Can you work these out from the model? Positions are in its coordinate system, mm. Face numbers are marked on the shaded views. A direction names the side the tool comes from. Give positions to 0.01 mm unless a question says otherwise; leave off trailing zeros. Order: outer loops, then holes, each group sorted by start corner. A loop starts at its lowest first (then second) coordinate and runs counter-clockwise, first axis right, second up. Notation, with made-up numbers: (9.25, 65.25) -> (49.25, 65.25) arc R18 cw to (49.25, 72.25) -> close; hole circle Ø4 at (89, -40). An arc over 180 degrees is marked (long way). Answer as CSV lines item,"result".
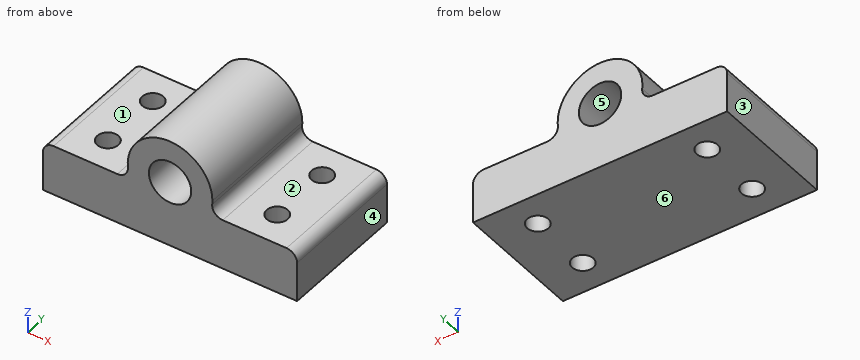
```python
from build123d import *

# Parameters (mm, degrees)
F0_R     = 25.4
F1_DEPTH = 152.4
F2_R     = 12.7
F3_DEPTH = 60.345965


with BuildPart() as f1:
    # F0 (on Front) → F1 (new body)
    with BuildSketch(Plane.XZ):
        with BuildLine():
            ThreePointArc((-50.585668, -4.661564), (-53.848843, -14.385271), (-63.232085, -18.526955))
            Line((-63.232085, -18.526955), (-139.7, -18.526955))
            ThreePointArc((-139.7, -18.526955), (-148.680256, -22.246699), (-152.4, -31.226955))
            Line((-152.4, -31.226955), (-152.4, -78.871921))
            Line((-152.4, -78.871921), (152.4, -78.871921))
            Line((152.4, -78.871921), (152.4, -31.226955))
            ThreePointArc((152.4, -31.226955), (148.680256, -22.246699), (139.7, -18.526955))
            Line((139.7, -18.526955), (63.232085, -18.526955))
            ThreePointArc((63.232085, -18.526955), (53.848843, -14.385271), (50.585668, -4.661564))
            ThreePointArc((50.585668, -4.661564), (0, -50.8), (-50.585668, -4.661564))
        make_face()
        with BuildLine():
            ThreePointArc((50.8, 0), (-2.333245, 50.746389), (-50.585668, -4.661564))
            ThreePointArc((-50.585668, -4.661564), (0, -50.8), (50.585668, -4.661564))
            ThreePointArc((50.585668, -4.661564), (50.746389, -2.333245), (50.8, 0))
        make_face()
        Circle(F0_R, mode=Mode.SUBTRACT)
    extrude(amount=F1_DEPTH)

    # F2 (on face) → F3 (cut, through all)
    with BuildSketch(Plane.XY.offset(-18.526955)):
        with Locations((-101.6, -38.1)):
            Circle(F2_R)
        with Locations((-101.6, -114.3)):
            Circle(F2_R)
        with Locations((101.6, -114.3)):
            Circle(F2_R)
        with Locations((101.6, -38.1)):
            Circle(F2_R)
    extrude(amount=-F3_DEPTH, mode=Mode.SUBTRACT)


solid = f1.part
```
Item 1: We'd pull the mould along Z, two halves only. Please class the marked faces 4, 5 and 6: released by +Z, released by -Z, zero draft, split by the parting line, or undercut.
Numbers:
face 4,"zero draft"
face 5,"undercut"
face 6,"released by -Z"
Item 2: Imagine slicing it at C-C, the plane x = -10.5. Please give me the cut outline in (y, z), then the cut area to 3 significant figures.
Numbers:
outline,"(-152.4, -78.87) -> (0, -78.87) -> (0, -23.13) -> (-152.4, -23.13) -> close; (-152.4, 23.13) -> (0, 23.13) -> (0, 49.7) -> (-152.4, 49.7) -> close"
area,"12,500 mm²"
Item 3: Imagine slicing it at D-D, the plane z = 6. Please give me the cut outline in (x, y).
Numbers:
outline,"(-50.44, -152.4) -> (-24.68, -152.4) -> (-24.68, 0) -> (-50.44, 0) -> close; (24.68, -152.4) -> (50.44, -152.4) -> (50.44, 0) -> (24.68, 0) -> close"
Item 4: Imagine slicing it at A-A, the plane x = -101.6. Please give me the cut outline in (y, z).
Numbers:
outline,"(-152.4, -78.87) -> (-127, -78.87) -> (-127, -18.53) -> (-152.4, -18.53) -> close; (-101.6, -78.87) -> (-50.8, -78.87) -> (-50.8, -18.53) -> (-101.6, -18.53) -> close; (-25.4, -78.87) -> (0, -78.87) -> (0, -18.53) -> (-25.4, -18.53) -> close"
Item 5: Please list where these lines run through material, in increasing order: line 1 along Y through (x, z) = (-101, -63); line 2 along Z through (x, y) = (0, -95); line 3 along Z through (x, y) = (-117, -145.5).
Numbers:
line 1,"y = -152.4 to -126.99, -101.61 to -50.79, -25.41 to 0"
line 2,"z = -78.87 to -25.4, 25.4 to 50.8"
line 3,"z = -78.87 to -18.53"
Item 6: For pin 1 (5 mm diameter, centred on x = 112.5, y = -122, fed in from +Z); pin 2 (12 mm diameter, centred on x = -49.5, y = -47, fed in from +Z); pin 3 (12 mm diameter, centred on y = -26, z = 21.5, fed in from -X), each with a flat end and sliding along its axis, tell me the tip position at first contact or that it passes through.
Numbers:
pin 1,"stops at z = -18.53"
pin 2,"stops at z = 26.24"
pin 3,"stops at x = -48.38"
Item 7: For the marked faces 1, 2 and 3, which set-ups out of +Z, -Z, +X, -X, +Y, -Y let a thin tool reach every point of the face, with its end or its side?
Numbers:
face 1,"+Z, -X, +Y, -Y"
face 2,"+Z, +X, +Y, -Y"
face 3,"+Z, -Z, -X, +Y, -Y"
Item 8: Imagine slicing it at B-B, the plane y = -38.1. Please give me the cut outline in (x, z).
Numbers:
outline,"(-152.4, -78.87) -> (-114.3, -78.87) -> (-114.3, -18.53) -> (-139.7, -18.53) arc R12.7 ccw to (-152.4, -31.23) -> close; (-88.9, -78.87) -> (88.9, -78.87) -> (88.9, -18.53) -> (63.23, -18.53) arc R12.7 cw to (50.59, -4.66) arc R50.8 ccw to (50.8, 0) arc R50.8 ccw (long way) to (-50.59, -4.66) arc R12.7 cw to (-63.23, -18.53) -> (-88.9, -18.53) -> close; (114.3, -78.87) -> (152.4, -78.87) -> (152.4, -31.23) arc R12.7 ccw to (139.7, -18.53) -> (114.3, -18.53) -> close; hole circle Ø50.8 at (0, 0)"
